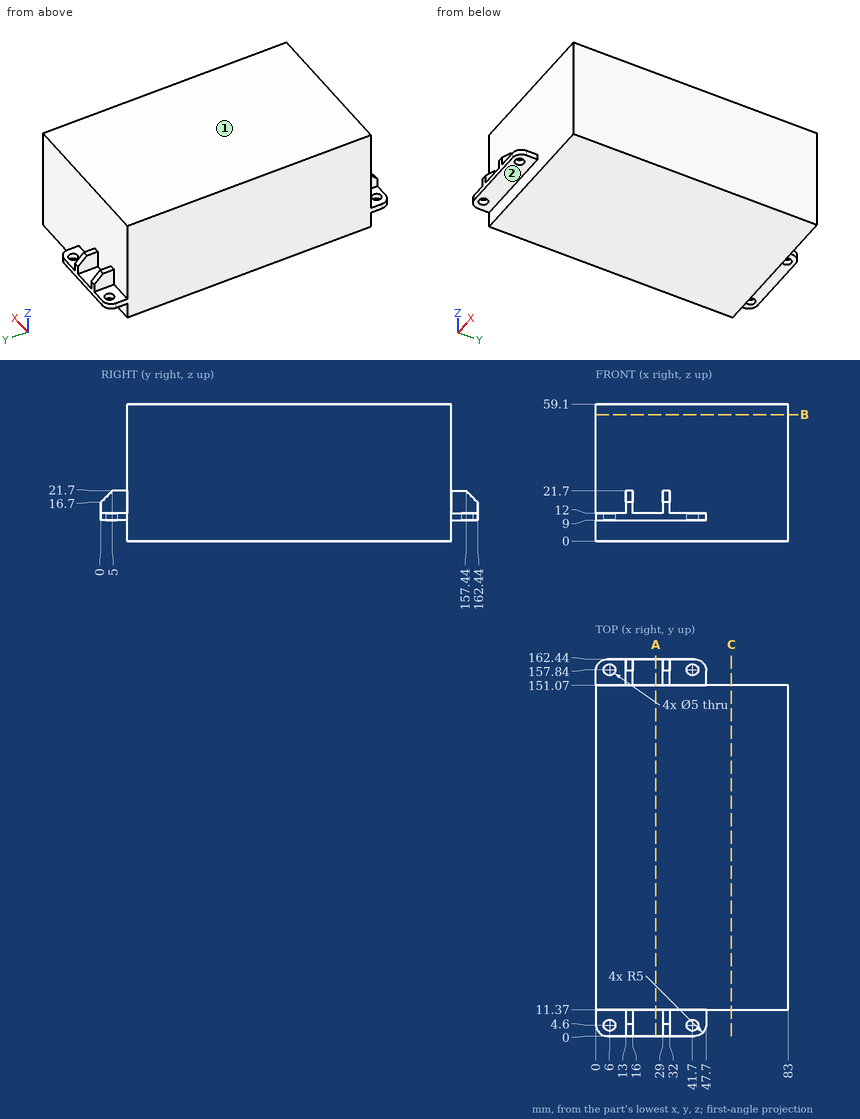
Study the drawing (mm; zero at the part's minimum x, y, z) and answer. A direction names the side the tool comes from. Round coordinates to 2 decimals unless told otherwise and drop trailing zeros. Write each loop counter-clockwise with the first axis right and the second up, starting at its lowest first coordinate (ties: lowest second). Pieces come first, ordered by that corner, then holes. Notation, with made-up numbers: (54, -32) -> (81, -32) arc R20 ccw to (81, -8) -> close; hole circle Ø11 at (-36.75, 56). An arc over 180 degrees is marked (long way). Write each question's results on one line, items separated by ' | '.
Item 1: Find the intervals of material crossed by line 1 along Y through (x, z) = (6, 10.45); line 2 along X through (y, z) = (157.84, 9.8); line 3 along X through (y, z) = (4, 11), in increasing order. Write a range as [from, to].
Result set:
line 1: [0, 2.1], [7.1, 155.34], [160.34, 162.44] | line 2: [0.02, 3.5], [8.5, 39.2], [44.2, 47.68] | line 3: [0.1, 3.57], [8.43, 39.27], [44.13, 47.6]
Item 2: A cutting plane is placed at B-B, the plane z = 54.5. Determine the outline of the cut face in (x, y), plus the area to 3 significant figures.
Result set:
outline: (0, 11.37) -> (83, 11.37) -> (83, 151.07) -> (0, 151.07) -> close | area: 11,600 mm^2
Item 3: A cutting plane is placed at A-A, the plane x = 26. Determine the outline of the cut face in (y, z).
Result set:
outline: (0, 9) -> (11.37, 9) -> (11.37, 0) -> (151.07, 0) -> (151.07, 9) -> (162.44, 9) -> (162.44, 12) -> (151.07, 12) -> (151.07, 59.1) -> (11.37, 59.1) -> (11.37, 12) -> (0, 12) -> close
Item 4: Flat-ended cylindrical pins translate along their axes: P1, Ø1.5, axis at y = 102.5, z = 10, coming from the -X side; P2, Ø1, axis at x = 25, z = 19.5, coming from the +Y side; P3, Ø6.5, axis at x = 41.7, y = 4.6, coming from the -Z side; P4, Ø1.5, axis at x = 30, y = 153, coming from the +Z side. Find the tip coordinate at first contact, or state that the pin passes through.
Result set:
P1: x = 0 | P2: y = 151.07 | P3: z = 9 | P4: z = 21.7
Item 5: A cutting plane is placed at C-C, the plane x = 58.5. Determine the outline of the cut face in (y, z), plus the area to 3 significant figures.
Result set:
outline: (11.37, 0) -> (151.07, 0) -> (151.07, 59.1) -> (11.37, 59.1) -> close | area: 8,260 mm^2
Item 6: Which of the six approach directions +Z, -Z, +X, -X, +Y, -Y give full straight-line access (tool end or side, diameter ignored) to the marked faces 1 and 2?
Result set:
face 1: +Z, +X, -X, +Y, -Y | face 2: -Z, +X, -X, -Y
